Geometry: final body of the model. Coordinates: model frame, mm. A direction names the side the tool comes from. Give positions to 0.01 mm unless a question says otherwise; leave off trailing zeros. Loops run counter-clockwise (first coordinate to the right, second up) from the corner with the lowest first, then second, coordinate; pieces in that order, holes last.
from build123d import *

# Parameters (mm, degrees)
SKETCH_1_R      = 2.55
EXTRUDE_1_DEPTH = 100


with BuildPart() as part:
    # 草图1 → 凸台-拉伸1 (new body)
    with BuildSketch(Plane.XY):
        with BuildLine():
            Line((-23.165408345, -6.388804564), (-23.165408345, -1.338804564))
            ThreePointArc((-23.165408345, -1.338804564), (-23.077540379, -1.12667253), (-22.865408345, -1.038804564))
            Line((-22.865408345, -1.038804564), (-22.665408345, -1.038804564))
            Line((-22.665408345, -1.038804564), (-22.665408345, -0.538804564))
            Line((-22.665408345, -0.538804564), (-21.165408345, -0.538804564))
            Line((-21.165408345, -0.538804564), (-21.165408345, -2.238804564))
            ThreePointArc((-21.165408345, -2.238804564), (-21.077540379, -2.450936598), (-20.865408345, -2.538804564))
            Line((-20.865408345, -2.538804564), (-19.665408345, -2.538804564))
            Line((-19.665408345, -2.538804564), (-17.651194783, -0.524591002))
            ThreePointArc((-17.651194783, -0.524591002), (-17.21764928, 0.124255696), (-17.065408345, 0.889622561))
            Line((-17.065408345, 0.889622561), (-17.065408345, 4.332768311))
            ThreePointArc((-17.065408345, 4.332768311), (-17.21764928, 5.098135176), (-17.651194783, 5.746981874))
            Line((-17.651194783, 5.746981874), (-19.665408345, 7.761195436))
            Line((-19.665408345, 7.761195436), (-20.865408345, 7.761195436))
            ThreePointArc((-20.865408345, 7.761195436), (-21.077540379, 7.67332747), (-21.165408345, 7.461195436))
            Line((-21.165408345, 7.461195436), (-21.165408345, 5.761195436))
            Line((-21.165408345, 5.761195436), (-22.665408345, 5.761195436))
            Line((-22.665408345, 5.761195436), (-22.665408345, 6.261195436))
            Line((-22.665408345, 6.261195436), (-22.865408345, 6.261195436))
            ThreePointArc((-22.865408345, 6.261195436), (-23.077540379, 6.349063402), (-23.165408345, 6.561195436))
            Line((-23.165408345, 6.561195436), (-23.165408345, 11.611195436))
            ThreePointArc((-23.165408345, 11.611195436), (-22.872515126, 12.318302217), (-22.165408345, 12.611195436))
            Line((-22.165408345, 12.611195436), (-17.115408345, 12.611195436))
            ThreePointArc((-17.115408345, 12.611195436), (-16.903276311, 12.52332747), (-16.815408345, 12.311195436))
            Line((-16.815408345, 12.311195436), (-16.815408345, 12.111195436))
            Line((-16.815408345, 12.111195436), (-16.315408345, 12.111195436))
            Line((-16.315408345, 12.111195436), (-16.315408345, 10.611195436))
            Line((-16.315408345, 10.611195436), (-18.015408345, 10.611195436))
            ThreePointArc((-18.015408345, 10.611195436), (-18.227540379, 10.52332747), (-18.315408345, 10.311195436))
            Line((-18.315408345, 10.311195436), (-18.315408345, 9.111195436))
            Line((-18.315408345, 9.111195436), (-16.301194783, 7.096981874))
            ThreePointArc((-16.301194783, 7.096981874), (-15.652348085, 6.663436371), (-14.88698122, 6.511195436))
            Line((-14.88698122, 6.511195436), (-11.44383547, 6.511195436))
            ThreePointArc((-11.44383547, 6.511195436), (-10.678468605, 6.663436371), (-10.029621907, 7.096981874))
            Line((-10.029621907, 7.096981874), (-8.015408345, 9.111195436))
            Line((-8.015408345, 9.111195436), (-8.015408345, 10.311195436))
            ThreePointArc((-8.015408345, 10.311195436), (-8.103276311, 10.52332747), (-8.315408345, 10.611195436))
            Line((-8.315408345, 10.611195436), (-10.015408345, 10.611195436))
            Line((-10.015408345, 10.611195436), (-10.015408345, 12.111195436))
            Line((-10.015408345, 12.111195436), (-9.515408345, 12.111195436))
            Line((-9.515408345, 12.111195436), (-9.515408345, 12.311195436))
            ThreePointArc((-9.515408345, 12.311195436), (-9.427540379, 12.52332747), (-9.215408345, 12.611195436))
            Line((-9.215408345, 12.611195436), (2.884591655, 12.611195436))
            ThreePointArc((2.884591655, 12.611195436), (3.096723689, 12.52332747), (3.184591655, 12.311195436))
            Line((3.184591655, 12.311195436), (3.184591655, 12.111195436))
            Line((3.184591655, 12.111195436), (3.684591655, 12.111195436))
            Line((3.684591655, 12.111195436), (3.684591655, 10.611195436))
            Line((3.684591655, 10.611195436), (1.984591655, 10.611195436))
            ThreePointArc((1.984591655, 10.611195436), (1.772459621, 10.52332747), (1.684591655, 10.311195436))
            Line((1.684591655, 10.311195436), (1.684591655, 9.111195436))
            Line((1.684591655, 9.111195436), (3.698805217, 7.096981874))
            ThreePointArc((3.698805217, 7.096981874), (4.347651915, 6.663436371), (5.11301878, 6.511195436))
            Line((5.11301878, 6.511195436), (8.55616453, 6.511195436))
            ThreePointArc((8.55616453, 6.511195436), (9.321531395, 6.663436371), (9.970378093, 7.096981874))
            Line((9.970378093, 7.096981874), (11.984591655, 9.111195436))
            Line((11.984591655, 9.111195436), (11.984591655, 10.311195436))
            ThreePointArc((11.984591655, 10.311195436), (11.896723689, 10.52332747), (11.684591655, 10.611195436))
            Line((11.684591655, 10.611195436), (9.984591655, 10.611195436))
            Line((9.984591655, 10.611195436), (9.984591655, 12.111195436))
            Line((9.984591655, 12.111195436), (10.484591655, 12.111195436))
            Line((10.484591655, 12.111195436), (10.484591655, 12.311195436))
            ThreePointArc((10.484591655, 12.311195436), (10.572459621, 12.52332747), (10.784591655, 12.611195436))
            Line((10.784591655, 12.611195436), (15.834591655, 12.611195436))
            ThreePointArc((15.834591655, 12.611195436), (16.541698436, 12.318302217), (16.834591655, 11.611195436))
            Line((16.834591655, 11.611195436), (16.834591655, 6.561195436))
            ThreePointArc((16.834591655, 6.561195436), (16.746723689, 6.349063402), (16.534591655, 6.261195436))
            Line((16.534591655, 6.261195436), (16.334591655, 6.261195436))
            Line((16.334591655, 6.261195436), (16.334591655, 5.761195436))
            Line((16.334591655, 5.761195436), (14.834591655, 5.761195436))
            Line((14.834591655, 5.761195436), (14.834591655, 7.461195436))
            ThreePointArc((14.834591655, 7.461195436), (14.746723689, 7.67332747), (14.534591655, 7.761195436))
            Line((14.534591655, 7.761195436), (13.334591655, 7.761195436))
            Line((13.334591655, 7.761195436), (11.320378093, 5.746981874))
            ThreePointArc((11.320378093, 5.746981874), (10.88683259, 5.098135176), (10.734591655, 4.332768311))
            Line((10.734591655, 4.332768311), (10.734591655, 0.889622561))
            ThreePointArc((10.734591655, 0.889622561), (10.88683259, 0.124255696), (11.320378093, -0.524591002))
            Line((11.320378093, -0.524591002), (13.334591655, -2.538804564))
            Line((13.334591655, -2.538804564), (14.534591655, -2.538804564))
            ThreePointArc((14.534591655, -2.538804564), (14.746723689, -2.450936598), (14.834591655, -2.238804564))
            Line((14.834591655, -2.238804564), (14.834591655, -0.538804564))
            Line((14.834591655, -0.538804564), (16.334591655, -0.538804564))
            Line((16.334591655, -0.538804564), (16.334591655, -1.038804564))
            Line((16.334591655, -1.038804564), (16.534591655, -1.038804564))
            ThreePointArc((16.534591655, -1.038804564), (16.746723689, -1.12667253), (16.834591655, -1.338804564))
            Line((16.834591655, -1.338804564), (16.834591655, -6.388804564))
            ThreePointArc((16.834591655, -6.388804564), (16.541698436, -7.095911345), (15.834591655, -7.388804564))
            Line((15.834591655, -7.388804564), (10.484591655, -7.388804564))
            Line((10.484591655, -7.388804564), (10.484591655, -6.888804564))
            Line((10.484591655, -6.888804564), (9.984591655, -6.888804564))
            Line((9.984591655, -6.888804564), (9.984591655, -5.388804564))
            Line((9.984591655, -5.388804564), (11.684591655, -5.388804564))
            ThreePointArc((11.684591655, -5.388804564), (11.896723689, -5.300936598), (11.984591655, -5.088804564))
            Line((11.984591655, -5.088804564), (11.984591655, -3.888804564))
            Line((11.984591655, -3.888804564), (9.970378093, -1.874591002))
            ThreePointArc((9.970378093, -1.874591002), (9.321531395, -1.441045499), (8.55616453, -1.288804564))
            Line((8.55616453, -1.288804564), (5.11301878, -1.288804564))
            ThreePointArc((5.11301878, -1.288804564), (4.347651915, -1.441045499), (3.698805217, -1.874591002))
            Line((3.698805217, -1.874591002), (1.684591655, -3.888804564))
            Line((1.684591655, -3.888804564), (1.684591655, -5.088804564))
            ThreePointArc((1.684591655, -5.088804564), (1.772459621, -5.300936598), (1.984591655, -5.388804564))
            Line((1.984591655, -5.388804564), (3.684591655, -5.388804564))
            Line((3.684591655, -5.388804564), (3.684591655, -6.888804564))
            Line((3.684591655, -6.888804564), (3.184591655, -6.888804564))
            Line((3.184591655, -6.888804564), (3.184591655, -7.088804564))
            ThreePointArc((3.184591655, -7.088804564), (3.096723689, -7.300936598), (2.884591655, -7.388804564))
            Line((2.884591655, -7.388804564), (-3.165408345, -7.388804564))
            Line((-3.165408345, -7.388804564), (-9.215408345, -7.388804564))
            ThreePointArc((-9.215408345, -7.388804564), (-9.427540379, -7.300936598), (-9.515408345, -7.088804564))
            Line((-9.515408345, -7.088804564), (-9.515408345, -6.888804564))
            Line((-9.515408345, -6.888804564), (-10.015408345, -6.888804564))
            Line((-10.015408345, -6.888804564), (-10.015408345, -5.388804564))
            Line((-10.015408345, -5.388804564), (-8.315408345, -5.388804564))
            ThreePointArc((-8.315408345, -5.388804564), (-8.103276311, -5.300936598), (-8.015408345, -5.088804564))
            Line((-8.015408345, -5.088804564), (-8.015408345, -3.888804564))
            Line((-8.015408345, -3.888804564), (-10.029621907, -1.874591002))
            ThreePointArc((-10.029621907, -1.874591002), (-10.678468605, -1.441045499), (-11.44383547, -1.288804564))
            Line((-11.44383547, -1.288804564), (-14.88698122, -1.288804564))
            ThreePointArc((-14.88698122, -1.288804564), (-15.652348085, -1.441045499), (-16.301194783, -1.874591002))
            Line((-16.301194783, -1.874591002), (-18.315408345, -3.888804564))
            Line((-18.315408345, -3.888804564), (-18.315408345, -5.088804564))
            ThreePointArc((-18.315408345, -5.088804564), (-18.227540379, -5.300936598), (-18.015408345, -5.388804564))
            Line((-18.015408345, -5.388804564), (-16.315408345, -5.388804564))
            Line((-16.315408345, -5.388804564), (-16.315408345, -6.888804564))
            Line((-16.315408345, -6.888804564), (-16.815408345, -6.888804564))
            Line((-16.815408345, -6.888804564), (-16.815408345, -7.088804564))
            ThreePointArc((-16.815408345, -7.088804564), (-16.903276311, -7.300936598), (-17.115408345, -7.388804564))
            Line((-17.115408345, -7.388804564), (-22.165408345, -7.388804564))
            ThreePointArc((-22.165408345, -7.388804564), (-22.872515126, -7.095911345), (-23.165408345, -6.388804564))
        make_face()
        with Locations((-13.165408345, 2.611195436)):
            Circle(SKETCH_1_R, mode=Mode.SUBTRACT)
        with Locations((6.834591655, 2.611195436)):
            Circle(SKETCH_1_R, mode=Mode.SUBTRACT)
        with BuildLine():
            Line((-9.265408345, 4.332768311), (-9.265408345, 0.889622561))
            ThreePointArc((-9.265408345, 0.889622561), (-9.11316741, 0.124255696), (-8.679621907, -0.524591002))
            Line((-8.679621907, -0.524591002), (-6.665408345, -2.538804564))
            Line((-6.665408345, -2.538804564), (-4.108301564, -5.095911345))
            ThreePointArc((-4.108301564, -5.095911345), (-3.783878215, -5.312684096), (-3.401194783, -5.388804564))
            Line((-3.401194783, -5.388804564), (-2.929621907, -5.388804564))
            ThreePointArc((-2.929621907, -5.388804564), (-2.546938475, -5.312684096), (-2.222515126, -5.095911345))
            Line((-2.222515126, -5.095911345), (0.334591655, -2.538804564))
            Line((0.334591655, -2.538804564), (2.348805217, -0.524591002))
            ThreePointArc((2.348805217, -0.524591002), (2.78235072, 0.124255696), (2.934591655, 0.889622561))
            Line((2.934591655, 0.889622561), (2.934591655, 4.332768311))
            ThreePointArc((2.934591655, 4.332768311), (2.78235072, 5.098135176), (2.348805217, 5.746981874))
            Line((2.348805217, 5.746981874), (0.334591655, 7.761195436))
            Line((0.334591655, 7.761195436), (-2.222515126, 10.318302217))
            ThreePointArc((-2.222515126, 10.318302217), (-2.546938475, 10.535074969), (-2.929621907, 10.611195436))
            Line((-2.929621907, 10.611195436), (-3.401194783, 10.611195436))
            ThreePointArc((-3.401194783, 10.611195436), (-3.783878215, 10.535074969), (-4.108301564, 10.318302217))
            Line((-4.108301564, 10.318302217), (-6.665408345, 7.761195436))
            Line((-6.665408345, 7.761195436), (-8.679621907, 5.746981874))
            ThreePointArc((-8.679621907, 5.746981874), (-9.11316741, 5.098135176), (-9.265408345, 4.332768311))
        make_face(mode=Mode.SUBTRACT)
    extrude(amount=EXTRUDE_1_DEPTH)


solid = part.part
Item 1: Draft query along Y for faces 1 (the face through (-21.165, 7, 49)), 2 (the face through (16.835, -4, 49)), 3 (the face through (13, -7.389, 49)). Return one class per face: +Y half, -Y half, draft (parallel to the pull), parting line (faces both ways), or undercut.
Values follow:
face 1: undercut
face 2: draft
face 3: -Y half
Item 2: Section query C-C on x = -0.5. Return loops of the section in (y, z), plus the area to 3 significant figures.
Values follow:
outline: (-7.39, 0) - (-3.37, 0) - (-3.37, 100) - (-7.39, 100) - close; (8.6, 0) - (12.61, 0) - (12.61, 100) - (8.6, 100) - close
area: 803 mm2
Item 3: Ray query, probe 1 along X at (y, z) = (-6, 35.5); probe 2 along X at (y, z) = (2.5, 29.5); probe 3 along Y at (x, z) = (-19, 58.5). Return the intervals inside material, ascending.
Values follow:
probe 1: x = -23.17 to -16.32, -10.02 to 3.68, 9.98 to 16.83
probe 2: x = -17.07 to -15.71, -10.62 to -9.27, 2.93 to 4.29, 9.38 to 10.73
probe 3: y = -7.39 to -1.87, 7.1 to 12.61
Item 4: Pin query (flat end, axial travel): pin 1 (3 mm diameter, centred on x = 7, z = 37.5, fed in from -Y); pin 2 (6 mm diameter, centred on x = -13.5, z = 81.5, fed in from +Y). Return the tip coordinate at first contact, or that it passes through.
Values follow:
pin 1: stops at y = -1.29
pin 2: stops at y = 12.11
Item 5: Set-up query: faces 4 (the face through (10.735, 3, 49)), 5 (the face through (-17.065, 3, 49)), 6 (the face through (-9.008, -2.896, 49.3)), 7 (the face through (7, -1.289, 49)). Return all of +Z, -Z, +X, -X, +Y, -Y with unobstructed straight access to the full face (end or side cutting, diameter ignored); none if empty.
Values follow:
face 4: +Z, -Z, +X
face 5: +Z, -Z, -X
face 6: +Z, -Z
face 7: +Z, -Z, -Y
Item 6: Section query A-A on x = 6. Return loops of the section in (y, z), plus the area to 3 significant figures.
Values follow:
outline: (-1.29, 0) - (0.2, 0) - (0.2, 100) - (-1.29, 100) - close; (5.02, 0) - (6.51, 0) - (6.51, 100) - (5.02, 100) - close
area: 298 mm2
Item 7: Section query B-B on z = 6. Give the number of separate pieces and of enclosed holes in the cut face, plus the area to 3 significant figures.
Values follow:
separate pieces: 1
enclosed holes: 3
area: 333 mm2
